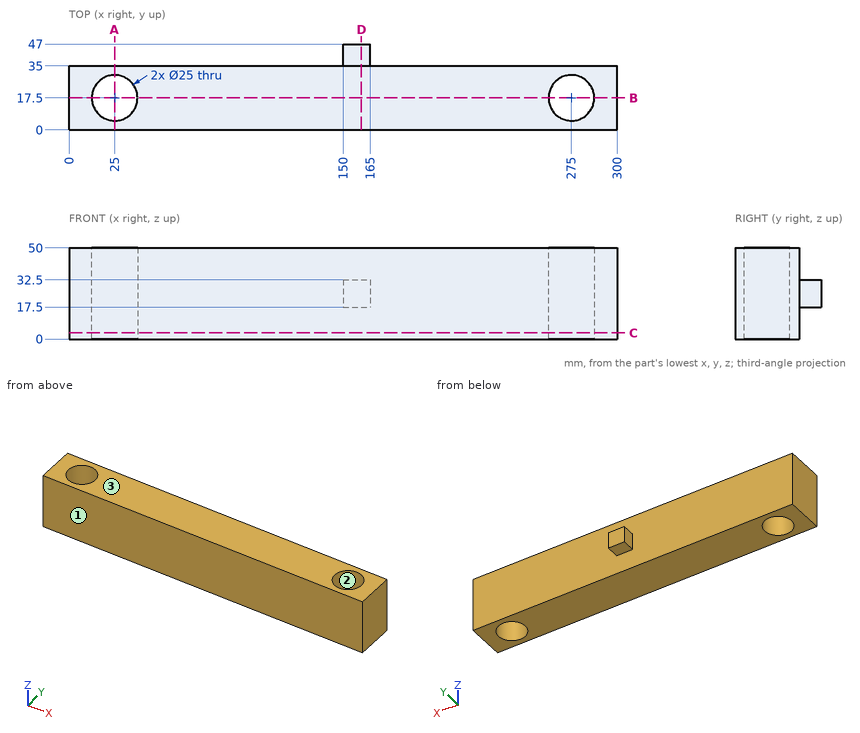
Geometry check sheet. Reference: drawing and pictorial views, mm from the part's lowest x, y, z. Give positions to 0.01 mm unless a question says otherwise; leave off trailing zeros. Loops run counter-clockwise (first coordinate to the right, second up) from the corner with the lowest first, then second, coordinate; pieces in that order, holes last. Notation, with made-up numbers: (-40, 68.5) - (-29, 68.5) arc R12 ccw to (-29, 90.5) - close; hole circle Ø5 at (76.5, -27). An arc over 180 degrees is marked (long way). Use CSV: the item, a comma, the result in double quotes. Start each with the question number.
Q1. Section check B-B, the plane y = 17.5. Record the cut outline in (x, z).
Q2. Section check C-C, the plane z = 3.5. Record the cut outline in (x, y), and give its area (3 significant figures).
Q3. Scan lines: probe 1 along X at (y, z) = (17, 23); probe 2 along Y at (x, z) = (275, 11); probe 3 along X at (y, z) = (19, 12). Record each from-to range of solid material in increasing order. Write a range as from..to.
Q4. Go/stop test with flat-tipped pins: pin 1 Ø3 at (x, z) = (200, 26.5) entering from +Y; pin 2 Ø3.5 at (x, y) = (161, 41) entering from +Z; pin 3 Ø6 at (y, z) = (43, 27) entering from +X. Record where each tip stops, or that it passes through.
Q5. Section check A-A, the plane x = 25. Record the cut outline in (y, z), and give its area (3 significant figures).
Q6. Release check for a two-part mould opening along Y. For the marked faces 1, 2 and 3 record: +Y half, -Y half, draft (parallel to the pull), parting line (faces both ways), or undercut.
Q7. Section check D-D, the plane x = 160. Record the cut outline in (y, z).
Findings below:
1,outline,"(0, 0) - (12.5, 0) - (12.5, 50) - (0, 50) - close; (37.5, 0) - (262.5, 0) - (262.5, 50) - (37.5, 50) - close; (287.5, 0) - (300, 0) - (300, 50) - (287.5, 50) - close"
2,outline,"(0, 0) - (300, 0) - (300, 35) - (0, 35) - close; hole circle Ø25 at (25, 17.5); hole circle Ø25 at (275, 17.5)"
2,area,"9,520 mm^2"
3,probe 1,"x = 0..12.51, 37.49..262.51, 287.49..300"
3,probe 2,"y = 0..5, 30..35"
3,probe 3,"x = 0..12.59, 37.41..262.59, 287.41..300"
4,pin 1,"stops at y = 35"
4,pin 2,"stops at z = 32.5"
4,pin 3,"stops at x = 165"
5,outline,"(0, 0) - (5, 0) - (5, 50) - (0, 50) - close; (30, 0) - (35, 0) - (35, 50) - (30, 50) - close"
5,area,"500 mm^2"
6,face 1,"-Y half"
6,face 2,"undercut"
6,face 3,"draft"
7,outline,"(0, 0) - (35, 0) - (35, 17.5) - (47, 17.5) - (47, 32.5) - (35, 32.5) - (35, 50) - (0, 50) - close"
